Build history of the part. All positions in model axes, mm. A direction names the side the tool comes from. Round coordinates to 2 decimals unless told otherwise and drop trailing zeros. Write each loop counter-clockwise with the first axis right and the second up, starting at its lowest first coordinate (ties: lowest second). Pieces come first, ordered by that corner, then holes. Notation, with made-up numbers: M 53.25,33 L 74.25,33 A34 cw 74.25,69 Z; hole C -5.5,67.25 d8. An arc over 180 degrees is marked long. One line per item, written item: value. Start each with the question number.
```python
from build123d import *

# Parameters (mm, degrees)
SKETCH1_W           = 58.1
SKETCH1_H           = 40.11
BOSS_EXTRUDE1_DEPTH = 80
SKETCH2_R           = 9.5
BOSS_EXTRUDE2_DEPTH = 2
SKETCH3_R           = 4
BOSS_EXTRUDE3_DEPTH = 15
SKETCH4_W           = 6.276876118
SKETCH4_H           = 1.998885949
CUT_EXTRUDE1_DEPTH  = 13
SKETCH5_R           = 3
BOSS_EXTRUDE4_DEPTH = 2
SKETCH6_R           = 2
CUT_EXTRUDE2_DEPTH  = 8
SKETCH7_R           = 4
CUT_EXTRUDE3_DEPTH  = 25.4


with BuildPart() as part:
    # Sketch1 → Boss-Extrude1 (new body)
    with BuildSketch(Plane.XY):
        with Locations((29.05, 20.055)):
            Rectangle(SKETCH1_W, SKETCH1_H)
    extrude(amount=BOSS_EXTRUDE1_DEPTH)

    # Sketch2 → Boss-Extrude2 (add)
    with BuildSketch(Plane.XY.offset(80)):
        with Locations((20.2, 20.055)):
            Circle(SKETCH2_R)
    extrude(amount=BOSS_EXTRUDE2_DEPTH)

    # Sketch3 → Boss-Extrude3 (add)
    with BuildSketch(Plane.XY.offset(82)):
        with Locations((20.2, 20.055)):
            Circle(SKETCH3_R)
    extrude(amount=BOSS_EXTRUDE3_DEPTH)

    # Sketch4 → Cut-Extrude1 (cut)
    with BuildSketch(Plane.XY.offset(97)):
        with Locations((20.2, 23.534403972)):
            Rectangle(SKETCH4_W, SKETCH4_H)
    extrude(amount=-CUT_EXTRUDE1_DEPTH, mode=Mode.SUBTRACT)

    # Sketch5 → Boss-Extrude4 (add)
    with BuildSketch(Plane.XY.offset(80)):
        with Locations((9.05, 34.055)):
            Circle(SKETCH5_R)
        with Locations((49.05, 34.055)):
            Circle(SKETCH5_R)
        with Locations((49.05, 6.055)):
            Circle(SKETCH5_R)
        with Locations((9.05, 6.055)):
            Circle(SKETCH5_R)
    extrude(amount=BOSS_EXTRUDE4_DEPTH)

    # Sketch6 → Cut-Extrude2 (cut)
    with BuildSketch(Plane.XY.offset(82)):
        with Locations((9.05, 34.055)):
            Circle(SKETCH6_R)
        with Locations((49.05, 34.055)):
            Circle(SKETCH6_R)
        with Locations((49.05, 6.055)):
            Circle(SKETCH6_R)
        with Locations((9.05, 6.055)):
            Circle(SKETCH6_R)
    extrude(amount=-CUT_EXTRUDE2_DEPTH, mode=Mode.SUBTRACT)

    # Sketch7 → Cut-Extrude3 (cut)
    with BuildSketch(Plane(origin=(58.1, 0, 0), x_dir=(0, 0, -1), z_dir=(1, 0, 0))):
        with Locations((-68.797911108, 20)):
            Circle(SKETCH7_R)
    extrude(amount=-CUT_EXTRUDE3_DEPTH, mode=Mode.SUBTRACT)


solid = part.part
```
Item 1: Cut at B-B, the plane x = 9.05. Write the cut outline in (y, z) (3 decimals).
Item 2: Cut at C-C, the plane y = 17.5. Write the cut outline in (x, z).
Item 3: Two-plate mould, pull along Y, no slides. Class faces 1 (the flat face through (0, 20, 39)), 2 (the cylindrical face through (50.958, 34.656, 78.056)), 3 (the flat face through (29, 25, 80)): pulls with the +Y half, pulls with the -Y half, needs draft (parallel to the pull), parting line crosses it, or undercut.
Item 4: Cut at D-D, the plane x = 20.2. Write the cut outline in (y, z) (3 decimals).
Item 5: Which spindle directions (+Z, -Z, +X, -X, +Y, -Y) get a long thin tool onto all of the face, cutting with end or side? Do faces 4 (the flat face through (20, 19, 97)), 5 (the cylindrical face through (50.9, 5.3, 78.1)), 6 (the flat face through (32.7, 20, 69)). Say none if no direction does.
Item 6: Cut at A-A, the plane x = 54.5. Write the cut outline in (y, z), plus the area to 3 significant figures.
Item 7: Drop flat-ended pins along their axis: pin 1 (3.5 mm diameter, centred on x = 49.05, y = 34.055, fed in from +Z); pin 2 (2 mm diameter, centred on x = 49.5, y = 35, fed in from +Z); pin 3 (1.9 mm diameter, centred on x = 20, z = 93, fed in from +Y). Give the stop position or say it passes through.
Item 8: Drill centre lines: line 1 (Y direction, x = 9.05, z = 78) (3 decimals); line 2 (Y direction, x = 9.05, z = 80.25) (3 decimals); line 3 (Z direction, x = 55, y = 4). Where is each one in solid material? Low to high.
Computed values:
1. outline: M 0,0 L 40.11,0 L 40.11,80 L 37.055,80 L 37.055,82 L 36.055,82 L 36.055,74 L 32.055,74 L 32.055,82 L 31.055,82 L 31.055,80 L 9.055,80 L 9.055,82 L 8.055,82 L 8.055,74 L 4.055,74 L 4.055,82 L 3.055,82 L 3.055,80 L 0,80 Z
2. outline: M 0,0 L 58.1,0 L 58.1,65.68 L 32.7,65.68 L 32.7,71.92 L 58.1,71.92 L 58.1,80 L 29.35,80 L 29.35,82 L 23.28,82 L 23.28,97 L 17.12,97 L 17.12,82 L 11.05,82 L 11.05,80 L 0,80 Z
3. face 1: needs draft
3. face 2: undercut
3. face 3: undercut
4. outline: M 0,0 L 40.11,0 L 40.11,80 L 29.555,80 L 29.555,82 L 24.055,82 L 24.055,84 L 22.535,84 L 22.535,97 L 16.055,97 L 16.055,82 L 10.555,82 L 10.555,80 L 0,80 Z
5. face 4: +Z, +X, -X, +Y, -Y
5. face 5: +Z
5. face 6: +X
6. outline: M 0,0 L 40.11,0 L 40.11,80 L 0,80 Z; hole C 20,68.8 d8
6. area: 3,160 mm2
7. pin 1: stops at z = 74
7. pin 2: stops at z = 82
7. pin 3: stops at y = 22.53
8. line 1: y = 0 to 4.055, 8.055 to 32.055, 36.055 to 40.11
8. line 2: y = 3.055 to 4.055, 8.055 to 9.055, 31.055 to 32.055, 36.055 to 37.055
8. line 3: z = 0 to 80
